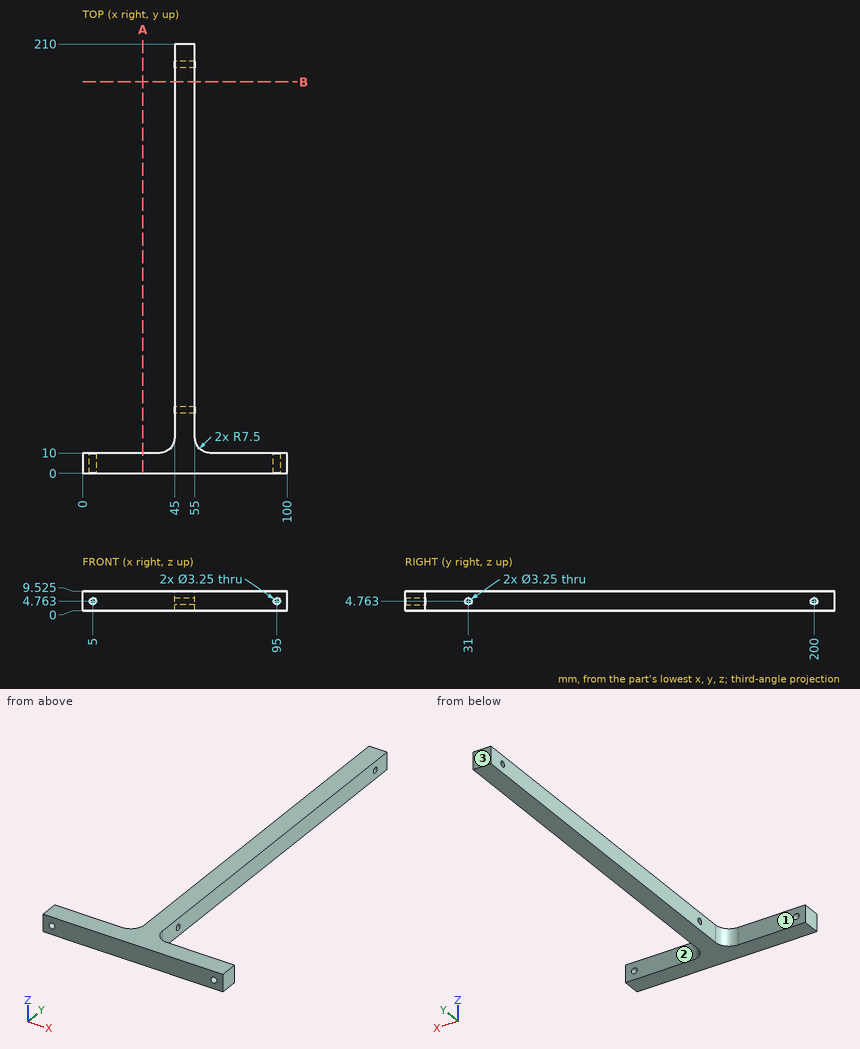
Study the drawing (mm; zero at the part's minimum x, y, z) and answer. A direction names the side the tool comes from. Coordinates: 2 decimals unless noted, no trailing zeros. Loops run counter-clockwise (first coordinate to the right, second up) from the corner with the lowest first, then second, coordinate; pieces in that order, holes last. Notation, with made-up numbers: (-11.5, -16.75) -> (40.5, -16.75) arc R27 ccw to (40.5, 1.25) -> close; hole circle Ø4 at (16, -20). An arc over 180 degrees is marked (long way). Write each question's results on one line, items separated by ' | '. Start each with the question number.
1) Consider line 1 along Y through (x, z) = (50.5, 4.25); line 2 along Y through (x, z) = (7, 7); line 3 along X through (y, z) = (131, 8). Determine where each line is inside the solid, lowest interval first.
2) Find section A-A on x = 29.5. Determine the outline of the cut face in (y, z) (1 decimal).
3) Find section B-B on y = 191.5. Determine the outline of the cut face in (x, z) (1 decimal).
4) Flat-ended cylindrical pins translate along their axes: P1, Ø1.5, axis at y = 115, z = 3.5, coming from the -X side; P2, Ø5, axis at y = 115, z = 3.5, coming from the +X side; P3, Ø2.5, axis at x = 95, z = 4.76, coming from the +Y side; P4, Ø5, axis at x = 81, z = 4, coming from the +Y side. Find the tip coordinate at first contact, or state that the pin passes through.
5) For the marked faces 1, 2 and 3, determine the directions among +Z, -Z, +X, -X, +Y, -Y from which every point of the face is accessible in a straight line to the end or side of a thin tool.
Response values:
1) line 1: y = 0 to 29.46, 32.54 to 198.46, 201.54 to 210 | line 2: y = 0 to 10 | line 3: x = 45 to 55
2) outline: (0, 0) -> (10, 0) -> (10, 9.5) -> (0, 9.5) -> close
3) outline: (45, 0) -> (55, 0) -> (55, 9.5) -> (45, 9.5) -> close
4) P1: stops at x = 45 | P2: stops at x = 55 | P3: passes through | P4: stops at y = 10
5) face 1: +Z, -Z, -X, +Y | face 2: +Z, -Z, +X, +Y | face 3: +Z, -Z, +X, -X, +Y
